Print and shaded views of the part. All mm, measured from the part's lowest x, y and z. A direction names the side the tool comes from. Round coordinates to 2 decimals unless told otherwise and drop trailing zeros. Loops run counter-clockwise (first coordinate to the right, second up) from the corner with the lowest first, then second, coordinate; pieces in that order, holes last. Notation, with made-up numbers: (-39, -20.5) - (4, -20.5) arc R30 ccw to (4, 4.5) - close; hole circle Ø8 at (-3.75, 74). An arc over 180 degrees is marked (long way). Use one line per item in the form item = value.
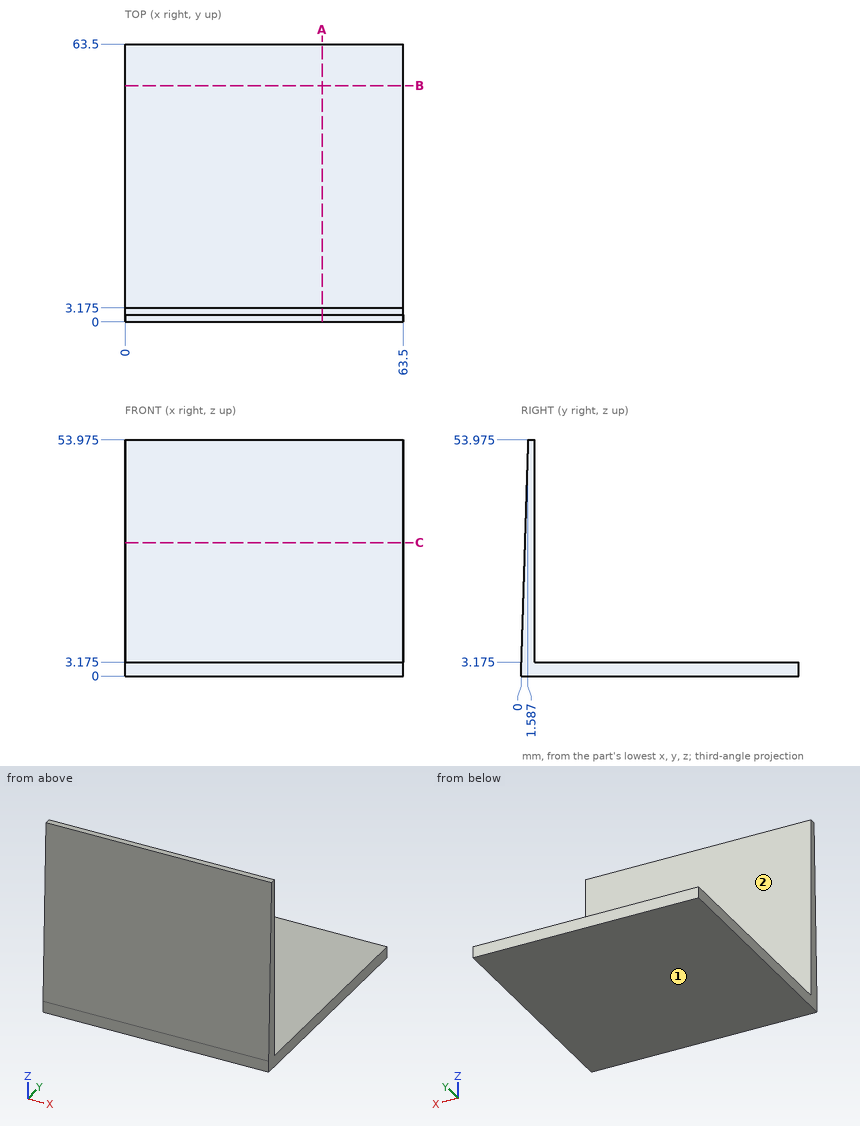
1. Flat gauge pins, fed straight in: pin 1 (6 mm diameter, centred on x = 33.5, z = 41.5, fed in from -Y); pin 2 (1 mm diameter, centred on x = 50.5, y = 55, fed in from +Z) (1 decimal); pin 3 (6 mm diameter, centred on x = 23.5, z = 46, fed in from -Y) (1 decimal). Where does each tip first touch, or does it go through?
Geometry check:
pin_1 = 1.1
pin_2 = 3.2
pin_3 = 1.2
2. Tool access for the marked faces 1 and 2: list every direction of +Z, -Z, +X, -X, +Y, -Y with a clear straight run to the whole face (end or side of a thin tool).
Geometry check:
face_1 = -Z, +X, -X, +Y, -Y
face_2 = +Z, +X, -X, +Y
3. Wall check: probe 1 along Z at (x, y) = (18, 41) (1 decimal); probe 2 along Y at (x, z) = (37, 10) (1 decimal); probe 3 along Y at (x, z) = (29, 17.5) (1 decimal). Give the ranges that are in metal, low to high.
Geometry check:
probe_1 = 0 to 3.2
probe_2 = 0.2 to 3.2
probe_3 = 0.4 to 3.2
4. Cut at B-B, the plane y = 54. Give the cut face in (x, z) (1 decimal).
Geometry check:
outline = (0, 0) - (63.5, 0) - (63.5, 3.2) - (0, 3.2) - close
5. Cut at C-C, the plane z = 30.5. Give the cut face in (x, y) (1 decimal).
Geometry check:
outline = (0, 0.9) - (63.5, 0.9) - (63.5, 3.2) - (0, 3.2) - close
6. Cut at A-A, the plane x = 45. Give the cut face in (y, z) (1 decimal).
Geometry check:
outline = (0, 0) - (63.5, 0) - (63.5, 3.2) - (3.2, 3.2) - (3.2, 54) - (1.6, 54) - (0, 3.2) - close
